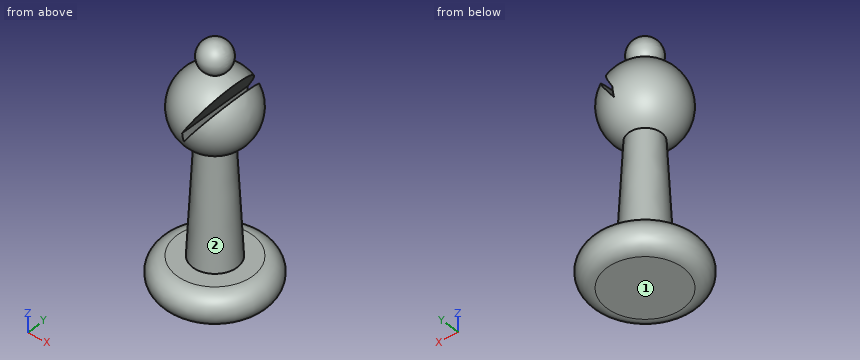
from build123d import *

# Parameters (mm, degrees)
PAD_DEPTH = 10


with BuildPart() as pad:
    # Sketch001 → Pad (new body, symmetric)
    with BuildSketch(Plane.XZ):
        Polygon((0, 26), (0, 27.5), (20, 62.141016), (20, 54.56296), align=None)
    extrude(amount=PAD_DEPTH, both=True)


with BuildPart() as cut001:
    # Sketch → Revolution (revolve)
    with BuildSketch(Plane.XZ):
        with BuildLine():
            Line((0, 0), (6, 0))
            ThreePointArc((6, 0), (8.5, 2.5), (6, 5))
            Line((6, 5), (0, 5))
            Line((0, 5), (0, 0))
        make_face()
        with BuildLine():
            Line((0, 5), (3.5, 5))
            Line((3.5, 5), (2.6, 22.592598))
            ThreePointArc((2.6, 22.592598), (5.966106, 28.63685), (1.4, 33.834381))
            ThreePointArc((1.4, 33.834381), (2.284564, 36.51911), (0, 38.18374))
            Line((0, 5), (0, 38.18374))
        make_face()
    revolve(axis=Axis((0, 0, 0), (0, 0, 1)))

    # Cut001: cut Pad
    add(pad.part, mode=Mode.SUBTRACT)


solid = cut001.part
Could you check a few things on this model? Use its own coordinates, in mm. Face numbers are marked on the shaded views. Give positions to 0.01 mm unless a question says otherwise; leave off trailing zeros. Write each loop counter-clockwise with the first axis right and the second up, starting at its lowest first coordinate (ties: lowest second). Pieces come first, ordered by that corner, then holes. Notation, with made-up numbers: (16.5, 60) -> (28.5, 60) arc R9 ccw to (28.5, 67) -> close; hole circle Ø5 at (28.25, 84.5). An arc over 180 degrees is marked (long way). Write each question's results on one line, items separated by ' | '. Start each with the question number.
Q1. I need wall thicknesses on probe 1 along X at (y, z) = (4, 27); probe 2 along Z at (x, y) = (-4, -1.5); probe 3 along Z at (x, y) = (6, -1.25). Which ranges of each line are inside material? Lowest first, please.
Q2. Suppose I cut it at B-B, the plane z = 28.5. List the corners of the cut face in (x, y) for me.
Q3. We'd pull the mould along Z, two halves only. Please class the marked faces 1 and 2: +Z half, -Z half, draft (parallel to the pull), parting line (faces both ways), or undercut.
Q4. Suppose I cut it at A-A, the plane z = 4. List the corners of the cut face in (x, y) for me, and give its area (3 significant figures).
Q5. Suppose I cut it at C-C, the plane z = 12.5. List the corners of the cut face in (x, y) for me, and give its area (3 significant figures).
Q6. I'm going to push flat-ended pins straight in: pin 1 Ø5 at (x, z) = (6.5, 11.5) entering from -Y; pin 2 Ø1 at (x, z) = (-2.5, 16.5) entering from -Y; pin 3 Ø1.2 at (y, z) = (1, 26.5) entering from +X; pin 4 Ø1.5 at (x, y) = (-3.5, 6.5) entering from +Z. Where does each tip first touch, or does it pass through?
Outcome:
1) probe 1: -4.36 to 0, 0.7 to 4.36 | probe 2: 0 to 5, 23.79 to 32.21 | probe 3: 0 to 5
2) outline: (0.58, -5.95) -> (0.58, 5.95) arc R5.98 ccw (long way) to start; (1.75, -5.72) arc R5.98 ccw to (1.75, 5.72) -> close
3) face 1: -Z half | face 2: undercut
4) outline: circle Ø16 at (0, 0) | area: 201 mm2
5) outline: circle Ø6.23 at (0, 0) | area: 30.5 mm2
6) pin 1: through | pin 2: y = -2.12 | pin 3: x = 5.88 | pin 4: z = 4.92
